Read the model definition and answer for the solid it produces. Units are mm, in the model's axes. A direction names the side the tool comes from. Round coordinates to 2 decimals unless told otherwise and drop trailing zeros. Order: outer loops, then holes, each group sorted by start corner. A loop starts at its lowest first (then second) coordinate and runs counter-clockwise, first axis right, second up. Notation, with made-up numbers: (58, 25) - (113, 25) arc R29 ccw to (113, 52) - close; hole circle Ø8 at (30.5, -40). An arc over 180 degrees is marked (long way). Put each result on its own line as item: value. Start each with the question number.
Q1. Section B-B on z = -5.5 is taken. Give the vertices of the cut face in (x, y), then the cut area to 3 significant figures.
Q2. Which of the six approach directions +Z, -Z, +X, -X, +Y, -Y give full straight-line access (tool end or side, diameter ignored) to faces 4 (the face through (16, 13, -21.964)), 5 (the face through (-23, 13, -21.964)), 6 (the face through (-6.026, 13, -4))?
Q3. Section C-C on y = 13.75 is taken. Give the vertices of the cut face in (x, z), then the cut area to 3 significant figures.
Q4. Section D-D on x = -8.5 is taken. Give the vertices of the cut face in (y, z).
Q5. Section A-A on x = -21.5 is taken. Give the vertices of the cut face in (y, z), then the cut area to 3 significant figures.
Q6. For a pull along Z with two mould halves and no side action, classify faces 1 (the face through (2.948, 13, -13)), 2 (the face through (13, 13, -18.957)), 3 (the face through (-28.349, 13, -20)) as pulls with the +Z half, pulls with the -Z half, needs draft (parallel to the pull), parting line crosses it, or undercut.
Q7. Each of these flat-tipped pins is pushed along its axis until it touches: pin 1 Ø13.5 at (x, y) = (-14, 8.5) entering from +Z; pin 2 Ø10 at (y, z) = (19.5, -10.5) entering from -X; pin 3 Ø14 at (y, z) = (16.5, -15) entering from +X; pin 4 Ø1.8 at (y, z) = (19, -23) entering from +X. Where does it stop, or does it pass through?
Q8. Find the intervals of material crossed by line 1 along Z through (x, y) = (13, 4.5); line 2 along X through (y, z) = (18, -25.5); line 3 along X through (y, z) = (9.75, -12.25), in increasing order. Write a range as from..to.
from build123d import *

# Parameters (mm, degrees)
BOSS_EXTRUDE2_DEPTH = 27


with BuildPart() as part:
    # Sketch2 → Boss-Extrude2 (new body)
    with BuildSketch(Plane(origin=(0, 0, 0), x_dir=(1, 0, 0), z_dir=(0, 1, 0))):
        with BuildLine():
            Line((-28.349494605, 21.964136687), (-17.349494605, 21.964136687))
            Line((-17.349494605, 21.964136687), (-17.349494605, 25.664136687))
            Line((-17.349494605, 25.664136687), (-28.349494605, 25.664136687))
            Line((-28.349494605, 25.664136687), (-28.349494605, 28.664136687))
            Line((-28.349494605, 28.664136687), (21.650505395, 28.664136687))
            Line((21.650505395, 28.664136687), (21.650505395, 25.664136687))
            Line((21.650505395, 25.664136687), (10.650505395, 25.664136687))
            Line((10.650505395, 25.664136687), (10.650505395, 21.964136687))
            Line((10.650505395, 21.964136687), (21.650505395, 21.964136687))
            Line((21.650505395, 21.964136687), (21.650505395, 18.957031621))
            Line((21.650505395, 18.957031621), (4.150505395, 18.957031621))
            Line((4.150505395, 18.957031621), (4.150505395, 6.457031621))
            ThreePointArc((4.150505395, 6.457031621), (-3.329004451, -0.970516956), (-10.847714263, 6.41734797))
            Line((-10.847714263, 6.41734797), (-6.026180838, 6.432389281))
            Line((-6.026180838, 6.432389281), (-4.222493535, 4.923226245))
            Line((-4.222493535, 4.923226245), (-4.222493535, 3.622157415))
            Line((-4.222493535, 3.622157415), (-6.026180838, 3.622157415))
            Line((-6.026180838, 3.622157415), (-6.026180838, 4.923226245))
            Line((-6.026180838, 4.923226245), (-9.437915177, 4.923226245))
            ThreePointArc((-9.437915177, 4.923226245), (-2.58302441, 0.278615253), (2.947813029, 6.440739557))
            Line((2.947813029, 6.440739557), (2.947813029, 18.957031621))
            Line((2.947813029, 18.957031621), (-28.349494605, 18.957031621))
            Line((-28.349494605, 18.957031621), (-28.349494605, 21.964136687))
        make_face()
    extrude(amount=BOSS_EXTRUDE2_DEPTH)


solid = part.part
Findings:
1. outline: (-10.78, 0) - (-4.91, 0) - (-4.91, 27) - (-10.78, 27) - close; (2.86, 0) - (4.08, 0) - (4.08, 27) - (2.86, 27) - close
1. area: 191 mm2
2. face 4: +X, +Y, -Y
2. face 5: -X, +Y, -Y
2. face 6: +Y, -Y
3. outline: (-28.35, -28.66) - (21.65, -28.66) - (21.65, -25.66) - (10.65, -25.66) - (10.65, -21.96) - (21.65, -21.96) - (21.65, -18.96) - (4.15, -18.96) - (4.15, -6.46) arc R7.5 ccw to (-10.85, -6.42) - (-6.03, -6.43) - (-4.22, -4.92) - (-4.22, -3.62) - (-6.03, -3.62) - (-6.03, -4.92) - (-9.44, -4.92) arc R6.3 cw to (2.95, -6.44) - (2.95, -18.96) - (-28.35, -18.96) - (-28.35, -21.96) - (-17.35, -21.96) - (-17.35, -25.66) - (-28.35, -25.66) - close
3. area: 454 mm2
4. outline: (0, -28.66) - (27, -28.66) - (27, -18.96) - (0, -18.96) - close; (0, -6.42) - (27, -6.42) - (27, -4.92) - (0, -4.92) - close; (0, -2.91) - (27, -2.91) - (27, -1.08) - (0, -1.08) - close
5. outline: (0, -28.66) - (27, -28.66) - (27, -25.66) - (0, -25.66) - close; (0, -21.96) - (27, -21.96) - (27, -18.96) - (0, -18.96) - close
5. area: 162 mm2
6. face 1: undercut
6. face 2: pulls with the +Z half
6. face 3: needs draft
7. pin 1: z = -0.12
7. pin 2: x = -10.85
7. pin 3: x = 21.65
7. pin 4: x = 10.65
8. line 1: -28.66..-25.66, -21.96..-18.96
8. line 2: -17.35..10.65
8. line 3: 2.95..4.15
